Solid Edge part; units mm, degrees
sketch "Sketch1" plane through (0, 0, 0) normal (0, 0, 1) x (1, 0, 0)
  circle A0 centre (0, 0) radius 9.135
extrude "Protrusion1" add sketch "Sketch1" along normal blind 9
sketch "Sketch2" plane through (0, 0, 9) normal (0, 0, 1) x (1, 0, 0)
  line L0 (0, -3.4641) -> (-3, -1.7321)
  line L1 (-3, -1.7321) -> (-3, 1.7321)
  line L2 (-3, 1.7321) -> (0, 3.4641)
  line L3 (0, 3.4641) -> (3, 1.7321)
  line L4 (3, 1.7321) -> (3, -1.7321)
  line L5 (3, -1.7321) -> (0, -3.4641)
extrude "Cutout1" cut sketch "Sketch2" against normal blind 4.5
sketch "Sketch3" plane through (0, 0, 0) normal (0, 0, -1) x (0, 1, 0)
  circle A0 centre (0, 0) radius 6
extrude "Protrusion2" add sketch "Sketch3" along normal blind 50
sketch "Sketch4" plane through (0, 0, -50) normal (0, 0, -1) x (0, 1, 0)
  circle A0 centre (0, 0) radius 5
extrude "Protrusion3" add sketch "Sketch4" along normal blind 16
chamfer "Chamfer1" distance 0.5 angle 45 1 edges at (0, -5, -66)
properties part number "156599"
Geometry check sheet. Reference: the model listing, model coordinates, mm. A direction names the side the tool comes from. Round coordinates to 2 decimals unless told otherwise and drop trailing zeros. Order: outer loops, then holes, each group sorted by start corner. A loop starts at its lowest first (then second) coordinate and runs counter-clockwise, first axis right, second up. Notation, with made-up numbers: M -12,81.5 L 18,81.5 A21 cw 18,117.5 Z; hole C 45,-37 d4. An arc over 180 degrees is marked long. Write item = value, one per line.
Q1. Release check for a two-part mould opening along Y. For faces 4 (the flat face through (1.5, 2.6, 6.8)), 5 (the flat face through (0, 0, -66)), 6 (the cylindrical face through (4.88, -1.08, -57.64)) record: released by +Y, released by -Y, zero draft, split by the parting line, or undercut.
Answer block:
face_4 = undercut
face_5 = zero draft
face_6 = split by the parting line
Q2. Set-up check for faces 1 (the flat face through (4, 0, 9)), 2 (the flat face through (3, 0, 7)), 3 (the flat face through (4, 4, -50)): record each of +Z, -Z, +X, -X, +Y, -Y from which the full face is reachable in a straight line by a thin tool's end or side.
Answer block:
face_1 = +Z, +X, -X, +Y, -Y
face_2 = +Z
face_3 = -Z
Q3. Section check B-B (z = -48). Enter the section's corners in (x, y), plus the area to 3 significant figures.
Answer block:
outline = C 0,0 d12
area = 113 mm^2
Q4. Section check A-A (y = 0). Enter the section's corners in (x, z) (3 decimals).
Answer block:
outline = M -9.135,0 L -6,0 L -6,-50 L -5,-50 L -5,-65.5 L -4.5,-66 L 4.5,-66 L 5,-65.5 L 5,-50 L 6,-50 L 6,0 L 9.135,0 L 9.135,9 L 3,9 L 3,4.5 L -3,4.5 L -3,9 L -9.135,9 Z
Q5. Section check C-C (y = 7.75). Enter the section's corners in (x, z).
Answer block:
outline = M -4.84,0 L 4.84,0 L 4.84,9 L -4.84,9 Z
Q6. Depth check by flat-ended pin: pin 1 Ø1.7 at (y, z) = (-1, 7) entering from +X; pin 2 Ø3 at (x, z) = (6, -30.5) entering from -Y; pin 3 Ø10 at (y, z) = (2.5, -7.5) entering from -X. Enter the tip coordinate at first touch or a pass-through.
Answer block:
pin_1 = 9.13
pin_2 = -3.97
pin_3 = -6
Q7. Scan lines: line 1 (Z direction, x = 0.5, y = 7.5); line 2 (Z direction, x = -4.5, y = 2.75); line 3 (Y direction, x = -0.25, z = -22). Record each from-to range of solid material in increasing order.
Answer block:
line_1 = 0 to 9
line_2 = -50 to 9
line_3 = -5.99 to 5.99
